For this review, take the finished solid that the model builds, in its own axes (mm). A direction names the side the tool comes from. Coordinates: 2 decimals unless noted, no trailing zeros. Order: outer loops, then holes, each group sorted by start corner. A loop starts at its lowest first (then second) coordinate and runs counter-clockwise, first axis right, second up. Notation, with made-up numbers: (-1, 87.25) - (36, 87.25) arc R29 ccw to (36, 119.25) - close; hole circle Ø11 at (41.25, 46). An arc over 180 degrees is marked (long way). One line per item, written item: value. Start each with the question number.
(1) For faces 1 (the flat face through (-10, 13, 7.982)), 2 (the flat face through (-10, 25, 5)), list the 3-axis set-ups (+Z, -Z, +X, -X, +Y, -Y) from which the entire face can be reached by the end or side of a thin tool; tool diameter is ignored.
(2) To check wall thickness, follow line 1 along Y through (x, z) = (11.75, 6); line 2 along Z through (x, y) = (130, 21); line 3 along Y through (x, z) = (-135.5, 8.5). State the ranges of each line that lie inside material, in increasing order.
(3) Consider section A-A on x = 44. Write out the cut boundary in (y, z).
(4) Clearance check with flat-ended pins moving along their axes: pin 1 (3 mm diameter, centred on y = 21, z = 3.75, fed in from -X); pin 2 (1.5 mm diameter, centred on x = -13.25, y = 12.5, fed in from +Z); pin 3 (2.5 mm diameter, centred on y = 4, z = 3.75, fed in from +X); pin 4 (4 mm diameter, centred on x = 37.5, y = 9.5, fed in from +Z). State where each tip first meets the part, or that it passes through.
(5) Consider section B-B on y = 8.75. Write out the cut boundary in (x, z), then the cut area to 3 significant figures.
Autodesk Inventor part; units mm, degrees
ref_plane "YZ Plane" through (0, 0, 0) normal (1, 0, 0) x (0, 1, 0)
ref_plane "XZ Plane" through (0, 0, 0) normal (0, 1, 0) x (-1, 0, 0)
ref_plane "XY Plane" through (0, 0, 0) normal (0, 0, 1) x (1, 0, 0)
sketch "Sketch1" plane through (0, 0, 0) normal (0, 0, 1) x (1, 0, 0)
  line L0 (127.75, 2.5629) -> (108.85, 2.5629) construction
  line L1 (-186.25, 0) -> (133.75, 0) construction
  line L2 (133.75, 0) -> (133.75, 5) construction
  line L3 (-186.25, 5) -> (133.75, 5) construction
  line L4 (-186.25, 0) -> (-186.25, 5) construction
  line L5 (133.75, 0) -> (-186.25, 0)
  line L6 (-186.25, 0) -> (-186.25, 25)
  line L7 (-186.25, 25) -> (133.75, 25)
  line L8 (133.75, 25) -> (133.75, 0)
  line L9 (-186.25, 0) -> (-186.25, 5)
  dimension "d1" = 25
extrude "Extrusion1" add sketch "Sketch1" along normal blind 9.9823
sketch "Sketch2" plane through (-186.25, 0, 0) normal (-1, 0, 0) x (0, 0, 1)
  line L0 (0, 0) -> (0, 25)
  line L1 (0, 0) -> (9.9823, 0)
  line L2 (9.9823, 25) -> (9.9823, 0)
  line L3 (0, 25) -> (9.9823, 25)
  point P0 (0, 0)
extrude "Extrusion2" cut sketch "Sketch2" against normal blind 36
sketch "Sketch3" plane through (0, 0, 9.9823) normal (0, 0, 1) x (1, 0, 0)
  line L0 (-157.75, 6.5) -> (141.25, 6.5)
  line L1 (141.25, 18.5) -> (-157.75, 18.5)
  line L2 (-150.25, 25) -> (-150.25, 0)
  line L3 (133.75, 0) -> (133.75, 25)
  line L4 (-150.25, 19) -> (133.75, 19)
  line L5 (133.75, 19) -> (133.75, 6)
  line L6 (133.75, 6) -> (-150.25, 6)
  line L7 (-150.25, 6) -> (-150.25, 19)
  point P0 (0, 0)
  dimension "d6" = 0.5
  dimension "d7" = 0.5
extrude "Extrusion3" cut sketch "Sketch3" against normal blind 2
sketch "Sketch4" plane through (133.75, 0, 0) normal (1, 0, 0) x (0, 0, -1)
  circle A0 centre (-3.7521, 4) radius 1.7
  circle A1 centre (-3.7521, 21) radius 1.7
  point P0 (0, 0)
hole "Hole1" at (133.75, 4, 3.7521) at (133.75, 21, 3.7521) direction (-1, 0, 0) diameter 3.242 depth 11.8
sketch "Sketch5" plane through (-150.25, 0, 0) normal (-1, 0, 0) x (0, 0, 1)
  circle A0 centre (3.7521, 21) radius 1.7
  circle A1 centre (3.7521, 4) radius 1.7
  point P0 (0, 0)
  point P1 (3.026, 2.4629)
  point P2 (3.026, 5.5371)
hole "Hole2" at (-150.25, 21, 3.7521) direction (1, 0, 0) diameter 3.242 depth 11.8
sketch "Sketch6" plane through (0, 0, 7.9823) normal (0, 0, 1) x (1, 0, 0)
  circle A0 centre (-138.25, 12.5) radius 1.7 construction
  circle A1 centre (-113.25, 12.5) radius 1.7 construction
  circle A2 centre (-88.25, 12.5) radius 1.75 construction
  circle A3 centre (-63.25, 12.5) radius 1.75 construction
  circle A4 centre (-38.25, 12.5) radius 1.75 construction
  circle A5 centre (-13.25, 12.5) radius 1.75 construction
  circle A6 centre (11.75, 12.5) radius 1.75 construction
  circle A7 centre (36.75, 12.5) radius 3 construction
  circle A8 centre (61.75, 12.5) radius 3 construction
  circle A9 centre (86.75, 12.5) radius 3 construction
  circle A10 centre (111.75, 12.5) radius 3 construction
  point P0 (0, 0)
hole "Hole3" at (-138.25, 12.5, 7.9823) at (-113.25, 12.5, 7.9823) at (-88.25, 12.5, 7.9823) at (-63.25, 12.5, 7.9823) at (-38.25, 12.5, 7.9823) at (-13.25, 12.5, 7.9823) at (11.75, 12.5, 7.9823) at (36.75, 12.5, 7.9823) at (61.75, 12.5, 7.9823) at (86.75, 12.5, 7.9823) at (111.75, 12.5, 7.9823) direction (0, 0, -1) diameter 2.459 end through all
properties part number "Y table support" material "Aluminum 6061"
Geometry check:
1. face 1: +Z, +X, -X
1. face 2: +Z, -Z, +X, -X, +Y
2. line 1: y = 0 to 11.27, 13.73 to 25
2. line 2: z = 0 to 2.13, 5.37 to 9.98
2. line 3: y = 0 to 6, 19 to 25
3. outline: (0, 0) - (25, 0) - (25, 9.98) - (19, 9.98) - (19, 7.98) - (6, 7.98) - (6, 9.98) - (0, 9.98) - close
4. pin 1: stops at x = -138.45
4. pin 2: passes through
4. pin 3: stops at x = 121.95
4. pin 4: stops at z = 7.98
5. outline: (-150.25, 0) - (133.75, 0) - (133.75, 7.98) - (-150.25, 7.98) - close
5. area: 2,270 mm^2
